from build123d import *

# Parameters (mm, degrees)
BOSS_EXTRUDE1_DEPTH      = 5
BOSS_EXTRUDE1_DEPTH_BACK = 5
SKETCH1_W                = 200
SKETCH1_H                = 160
SKETCH2_R                = 5
SKETCH2_R_2              = 2.1
CUT_EXTRUDE1_DEPTH       = 257.32011236


with BuildPart() as part:
    # Sketch1 → Boss-Extrude1 (new, two sides: drawn at the far end of the back side and taken through both)
    with BuildSketch(Plane(origin=(0, 0, 0), x_dir=(1, 0, 0), z_dir=(0, 1, 0)).offset(-BOSS_EXTRUDE1_DEPTH_BACK)):
        with Locations((100, 80)):
            Rectangle(SKETCH1_W, SKETCH1_H)
    extrude(amount=BOSS_EXTRUDE1_DEPTH + BOSS_EXTRUDE1_DEPTH_BACK)

    # Sketch2 → Cut-Extrude1 (cut, through all)
    with BuildSketch(Plane(origin=(0, 5, 0), x_dir=(1, 0, 0), z_dir=(0, 1, 0))):
        with Locations(Location((180, 150, 0), (0, 0, 270))):
            Circle(SKETCH2_R)
        with Locations(Location((74.197673555, 105.802326445, 0), (0, 0, 270))):
            Circle(SKETCH2_R_2)
        with Locations(Location((74.197673555, 54.197673555, 0), (0, 0, 270))):
            Circle(SKETCH2_R_2)
        with Locations(Location((125.802326445, 54.197673555, 0), (0, 0, 270))):
            Circle(SKETCH2_R_2)
        with Locations(Location((125.802326445, 105.802326445, 0), (0, 0, 270))):
            Circle(SKETCH2_R_2)
        with Locations(Location((180, 10, 0), (0, 0, 270))):
            Circle(SKETCH2_R)
        with Locations(Location((20, 10, 0), (0, 0, 270))):
            Circle(SKETCH2_R)
        with Locations(Location((20, 150, 0), (0, 0, 270))):
            Circle(SKETCH2_R)
    extrude(amount=-CUT_EXTRUDE1_DEPTH, mode=Mode.SUBTRACT)


solid = part.part
Geometry: final body of the model. Coordinates: model frame, mm. Coordinates: 2 decimals unless noted, no trailing zeros. Order: outer loops, then holes, each group sorted by start corner. A loop starts at its lowest first (then second) coordinate and runs counter-clockwise, first axis right, second up. Notation, with made-up numbers: M -25.75,16 L 29.25,16 A34 cw 29.25,53 Z; hole C 25.25,-20.75 d3. An arc over 180 degrees is marked long. One line per question, with ' | ' between items. Start each with the question number.
Item 1: Cut plane A-A, the plane z = -150. Return the cut outline in (x, y), then the cut area to 3 significant figures.
Item 2: Draft query along X for faces 1 (the flat face through (99, 0, -160)), 2 (the cylindrical face through (72.148, 0.07, -54.653)), 3 (the flat face through (200, 0, -79)), 4 (the cylindrical face through (184.957, 0.07, -150.651)). Return one class per face: released by +X, released by -X, zero draft, split by the parting line, or undercut.
Item 3: Ray query, probe 1 along X at (y, z) = (1.25, -10); probe 2 along Z at (x, y) = (124, 3); probe 3 along Z at (x, y) = (73.5, -4). Return the intervals inside material, ascending. Write a range as [from, to].
Item 4: Cut plane B-B, the plane x = 180. Return the cut outline in (y, z).
Item 5: Pin query (flat end, axial travel): pin 1 Ø2.5 at (x, z) = (125.8, -54.2) entering from -Y; pin 2 Ø13 at (x, z) = (20, -150) entering from -Y. Return the tip coordinate at first contact, or that it passes through.
A:
1) outline: M 0,-5 L 15,-5 L 15,5 L 0,5 Z; M 25,-5 L 175,-5 L 175,5 L 25,5 Z; M 185,-5 L 200,-5 L 200,5 L 185,5 Z | area: 1,800 mm2
2) face 1: zero draft | face 2: undercut | face 3: released by +X | face 4: undercut
3) probe 1: x = [0, 15], [25, 175], [185, 200] | probe 2: z = [-160, -106.88], [-104.72, -55.28], [-53.12, 0] | probe 3: z = [-160, -107.78], [-103.82, -56.18], [-52.22, 0]
4) outline: M -5,-160 L 5,-160 L 5,-155 L -5,-155 Z; M -5,-145 L 5,-145 L 5,-15 L -5,-15 Z; M -5,-5 L 5,-5 L 5,0 L -5,0 Z
5) pin 1: passes through | pin 2: stops at y = -5
